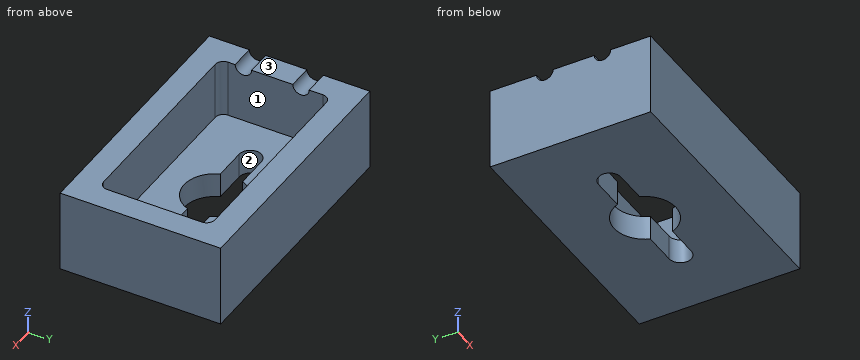
Autodesk Inventor part; units mm, degrees
ref_plane "YZ Plane" through (0, 0, 0) normal (1, 0, 0) x (0, 1, 0)
ref_plane "XZ Plane" through (0, 0, 0) normal (0, 1, 0) x (-1, 0, 0)
ref_plane "XY Plane" through (0, 0, 0) normal (0, 0, 1) x (1, 0, 0)
sketch "Skizze1" plane through (0, 0, 0) normal (0, 0, 1) x (1, 0, 0)
  line L0 (0, 22.5879) -> (0, -19.7685)
  line L1 (-28.9042, 0) -> (30.2947, 0)
  line L2 (-15.85, 9.75) -> (15.85, 9.75)
  line L3 (15.85, 9.75) -> (15.85, -9.75)
  line L4 (15.85, -9.75) -> (-15.85, -9.75)
  line L5 (-15.85, -9.75) -> (-15.85, 9.75)
  point P0 (0, 0)
  dimension "d0" = 31.7
  dimension "d1" = 19.5
extrude "Extrusion1" add sketch "Skizze1" along normal blind 10
sketch "Skizze2" plane through (0, 0, 10) normal (0, 0, 1) x (1, 0, 0)
  line L0 (-12.85, 6.75) -> (12.85, 6.75)
  line L1 (12.85, 6.75) -> (12.85, -6.75)
  line L2 (12.85, -6.75) -> (-12.85, -6.75)
  line L3 (-12.85, -6.75) -> (-12.85, 6.75)
  line L4 (15.85, -9.75) -> (15.85, 9.75)
  line L5 (-15.85, -9.75) -> (15.85, -9.75)
  line L6 (-15.85, 9.75) -> (-15.85, -9.75)
  line L7 (15.85, 9.75) -> (-15.85, 9.75)
  point P0 (0, 0)
  dimension "d4" = 3
  dimension "d5" = 3
  dimension "d6" = 3
  dimension "d7" = 3
extrude "Extrusion2" cut sketch "Skizze2" against normal blind 7 contours L0 L1 L2 L3
sketch "Skizze3" plane through (-15.85, -9.75, 0) normal (-1, 0, 0) x (0, 0, 1)
  line L0 (10, 0) -> (10, 19.5)
  arc A0 (10, 13.8534) -> (10, 11.8534) centre (10, 12.8534) ccw
  arc A1 (10, 6.8534) -> (10, 4.8534) centre (10, 5.8534) ccw
  line L1 (10, 19.5) -> (10, 0)
  line L2 (-1.0357, 9.3534) -> (13.3763, 9.3534)
  point P0 (0, 9.75)
  dimension "d10" = 7
  dimension "d11" = 1
  dimension "d12" = 1
extrude "Extrusion3" cut sketch "Skizze3" against normal blind 7
fillet "Rundung1" radius 1 4 edges at (12.85, -6.75, 6.5) (12.85, 6.75, 6.5) (-12.85, 6.75, 6.5) (-12.85, -6.75, 6.5)
sketch "Skizze4" plane through (0, 0, 3) normal (0, 0, 1) x (1, 0, 0)
  arc A0 (12.85, 5.75) -> (11.85, 6.75) centre (11.85, 5.75) ccw
  line L0 (11.85, 6.75) -> (-11.85, 6.75)
  arc A1 (-11.85, 6.75) -> (-12.85, 5.75) centre (-11.85, 5.75) ccw
  line L1 (-12.85, 5.75) -> (-12.85, -5.75)
  arc A2 (-12.85, -5.75) -> (-11.85, -6.75) centre (-11.85, -5.75) ccw
  line L2 (-11.85, -6.75) -> (11.85, -6.75)
  arc A3 (11.85, -6.75) -> (12.85, -5.75) centre (11.85, -5.75) ccw
  line L3 (12.85, -5.75) -> (12.85, 5.75)
  line L4 (15.85, 9.75) -> (15.85, -9.75)
  line L5 (15.85, -9.75) -> (-15.85, -9.75)
  line L6 (-15.85, -9.75) -> (-15.85, 9.75)
  line L7 (-15.85, 9.75) -> (15.85, 9.75)
  circle A4 centre (-7.5, 0) radius 2.5
  circle A5 centre (7.5, 0) radius 2.5
  circle A6 centre (-7.5, 0) radius 1.35
  circle A7 centre (7.5, 0) radius 1.35
  circle A8 centre (0, 0) radius 3.75
  circle A9 centre (0, 0) radius 1.35
  line L8 (-7.5, 1.35) -> (0, 1.35)
  line L9 (-7.5, -1.35) -> (0, -1.35)
  line L10 (0, 1.35) -> (7.5, 1.35)
  line L11 (7.5, -1.35) -> (0, -1.35)
  dimension "d16" = 7.5
  dimension "d17" = 7.5
  dimension "d18" = 5
  dimension "d19" = 5
  dimension "d20" = 2.7
  dimension "d21" = 2.7
  dimension "d22" = 7.5
  dimension "d23" = 2.7
extrude "Extrusion4" cut sketch "Skizze4" against normal blind 5 contours A4 L9 A6 L8 | A4 L8 A8 L9 | A6 | L8 A9 L9 A8 | A8 L10 L8 | L9 L11 A8 | L10 A5 L11 A8 | A8 L11 A9 L10 | A9 | L10 A7 L11 A5 | A7 picked at (-5.3984, -0.1575) picked at (5.3974, -0.0542)
properties part number "ls-halterung"
Verification items for the finished model (mm, model axes). Face numbers are marked on the shaded views. A direction names the side the tool comes from. Give positions to 0.01 mm unless a question says otherwise; leave off trailing zeros. Loops run counter-clockwise (first coordinate to the right, second up) from the corner with the lowest first, then second, coordinate; pieces in that order, holes last.
1. Section check B-B, the plane y = 0. Enter the section's corners in (x, z), then the cut area to 3 significant figures.
2. Thickness scan on line 1 (X direction, y = -0.5, z = 7.25); line 2 (Y direction, x = 11, z = 5); line 3 (Z direction, x = 0, y = 4.25). Record the ranges inside material, lowest first.
3. Section check A-A, the plane x = 6.5. Enter the section's corners in (y, z).
4. Section check C-C, the plane z = 4. Enter the section's corners in (x, y).
5. Section check D-D, the plane y = -4.5. Enter the section's corners in (x, z).
6. Go/stop test with a flat-tipped pin: pin 1 Ø4 at (x, y) = (-2, -3.5) entering from +Z. Record where the tip stops, or that it passes through.
7. Set-up check for the marked faces 1, 2 and 3: record each of +Z, -Z, +X, -X, +Y, -Y from which the full face is reachable in a straight line by a thin tool's end or side.
Geometry says:
1. outline: (-15.85, 0) - (-8.85, 0) - (-8.85, 3) - (-12.85, 3) - (-12.85, 10) - (-15.85, 10) - close; (8.85, 0) - (15.85, 0) - (15.85, 10) - (12.85, 10) - (12.85, 3) - (8.85, 3) - close
1. area: 84.0 mm2
2. line 1: x = -15.85 to -12.85, 12.85 to 15.85
2. line 2: y = -9.75 to -6.75, 6.75 to 9.75
2. line 3: z = 0 to 3
3. outline: (-9.75, 0) - (-1.35, 0) - (-1.35, 3) - (-6.75, 3) - (-6.75, 10) - (-9.75, 10) - close; (1.35, 0) - (9.75, 0) - (9.75, 10) - (6.75, 10) - (6.75, 3) - (1.35, 3) - close
4. outline: (-15.85, -9.75) - (15.85, -9.75) - (15.85, 9.75) - (-15.85, 9.75) - close; hole (-12.85, -5.75) arc R1 ccw to (-11.85, -6.75) - (11.85, -6.75) arc R1 ccw to (12.85, -5.75) - (12.85, 5.75) arc R1 ccw to (11.85, 6.75) - (-11.85, 6.75) arc R1 ccw to (-12.85, 5.75) - close
5. outline: (-15.85, 0) - (15.85, 0) - (15.85, 10) - (12.85, 10) - (12.85, 3) - (-12.85, 3) - (-12.85, 9.2) - (-15.85, 9.2) - close
6. pin 1: stops at z = 3
7. face 1: +Z
7. face 2: +Z, -Z
7. face 3: +Z, +X, -X, +Y, -Y
